The model under review builds one solid part; all positions refer to its coordinate system, in mm. A direction names the side the tool comes from. Round coordinates to 2 decimals unless told otherwise and drop trailing zeros. Order: outer loops, then holes, each group sorted by start corner. A loop starts at its lowest first (then second) coordinate and runs counter-clockwise, first axis right, second up. Notation, with made-up numbers: M 74,55 L 80,55 A22 cw 80,71 Z; hole C 44,87.5 d3. An arc over 180 degrees is marked long. Use a Markdown table: item, result. Add a question column.
1. Consider section D-D on z = 28.5. State the section outline as (x, y) points.
2. Consider section C-C on x = 7.5. State the section outline as (y, z) points, then the cut area to 3 significant figures.
3. To check wall thickness, follow probe 1 along X at (y, z) = (5.5, 7); probe 2 along Y at (x, z) = (7.5, 7); probe 3 along Y at (x, z) = (7.5, 7.5). State the ranges of each line that lie inside material, in increasing order.
4. The part is to be moulded in two halves that separate along Y. For faces 1 (the flat face through (7, 0, 15)), 2 (the flat face through (5.7, 9.3, 0)), 3 (the cylindrical face through (6.633, 9.405, 4.93)), say which applies: +Y half, -Y half, draft (parallel to the pull), parting line (faces both ways), or undercut.
5. Insertion check: P1, Ø2, axis at x = 4, y = 11, coming from the -Z side; P2, Ø3, axis at x = 6, y = 9.5, coming from the +Z side; P3, Ø8, axis at x = 11.5, y = 5, coming from the +Z side; P4, Ø6.5, axis at x = 7.5, y = 5.5, coming from the +Z side. Each pin has a flat end and moves straight along its axis. Give the tip position at first contact, or say it passes through.
6. Consider section B-B on z = 3. State the section outline as (x, y) points, then the cut area to 3 significant figures.
7. For faces 4 (the flat face through (0, 6, 11)), 5 (the flat face through (7, 5, 10)), list the 3-axis set-ups (+Z, -Z, +X, -X, +Y, -Y) from which the entire face can be reached by the end or side of a thin tool; tool diameter is ignored.
8. Consider section A-A on y = 5.5. State the section outline as (x, z) points, then the cut area to 3 significant figures.
from build123d import *

# Parameters (mm, degrees)
F0_W     = 15
F0_H     = 15
F1_DEPTH = 30
F3_DEPTH = 25
F4_R     = 4
F5_DEPTH = 10


# Not quite as in the source:
# - a feature names something its author has since deleted; it is built from what else it names


with BuildPart() as f1:
    # F0 (on Top) → F1 (new body)
    with BuildSketch(Plane.XY):
        with Locations((7.5, 7.5)):
            Rectangle(F0_W, F0_H)
    extrude(amount=F1_DEPTH)

    # F2 (on face) → F3 (cut)
    with BuildSketch(Plane.YZ.offset(15)):
        Polygon((15, 30), (0, 30), (15, 0), align=None)
    extrude(amount=-F3_DEPTH, mode=Mode.SUBTRACT)

    # F4 (on face) → F5 (cut)
    with BuildSketch(Plane(origin=(0, 0, 0), x_dir=(1, 0, 0), z_dir=(0, 0, -1))):
        with Locations((7.5, -5.5)):
            Circle(F4_R)
    extrude(amount=-F5_DEPTH, mode=Mode.SUBTRACT)


solid = f1.part
Answer block:
| question | item | result |
|---|---|---|
| 1 | outline | M 0,0 L 15,0 L 15,0.75 L 0,0.75 Z |
| 2 | outline | M 0,0 L 1.5,0 L 1.5,10 L 9.5,10 L 9.5,0 L 15,0 L 0,30 Z |
| 2 | area | 145 mm^2 |
| 3 | probe 1 | 0 to 3.5, 11.5 to 15 |
| 3 | probe 2 | 0 to 1.5, 9.5 to 11.5 |
| 3 | probe 3 | 0 to 1.5, 9.5 to 11.25 |
| 4 | face 1 | -Y half |
| 4 | face 2 | draft |
| 4 | face 3 | undercut |
| 5 | P1 | z = 0 |
| 5 | P2 | z = 14 |
| 5 | P3 | z = 28 |
| 5 | P4 | z = 25.5 |
| 6 | outline | M 0,0 L 15,0 L 15,13.5 L 0,13.5 Z; hole C 7.5,5.5 d8 |
| 6 | area | 152 mm^2 |
| 7 | face 4 | +Z, -Z, -X, +Y, -Y |
| 7 | face 5 | -Z |
| 8 | outline | M 0,0 L 3.5,0 L 3.5,10 L 11.5,10 L 11.5,0 L 15,0 L 15,19 L 0,19 Z |
| 8 | area | 205 mm^2 |
